Can you work these out from the model? Positions are in its coordinate system, mm. Face numbers are marked on the shaded views. A direction names the side the tool comes from. Give positions to 0.01 mm unless a question says otherwise; leave off trailing zeros. Order: outer loops, then holes, each group sorted by start corner. A loop starts at its lowest first (then second) coordinate and runs counter-clockwise, first axis right, second up. Notation, with made-up numbers: (-18, 28.5) - (8, 28.5) arc R33 cw to (8, 61.5) - close; hole circle Ø1 at (-26, 10). An arc over 180 degrees is marked (long way). Answer as CSV lines item,"result".
```python
from build123d import *

# Parameters (mm, degrees)
BOSS_EXTRUDE1_DEPTH = 8.636


with BuildPart() as part:
    # Sketch1 → Revolve1 (revolve)
    with BuildSketch(Plane.XY):
        Polygon((0, 0), (0, 29.972), (6.477, 29.972), (6.477, 38.354), (11.1125, 38.354), (11.1125, 0), (11.1125, -27.432), (4.5125, -27.432), (4.5125, -8.636), (0, -8.636), align=None)
    revolve(axis=Axis((11.1125, 38.354, 0), (0, -1, 0)))

    # Sketch2 → Boss-Extrude1 (add)
    with BuildSketch(Plane.XZ.offset(8.636)):
        Polygon((23.944109733, 0), (17.528304866, 11.1125), (4.696695134, 11.1125), (-1.719109733, 0), (4.696695134, -11.1125), (17.528304866, -11.1125), align=None)
    extrude(amount=-BOSS_EXTRUDE1_DEPTH)


solid = part.part
```
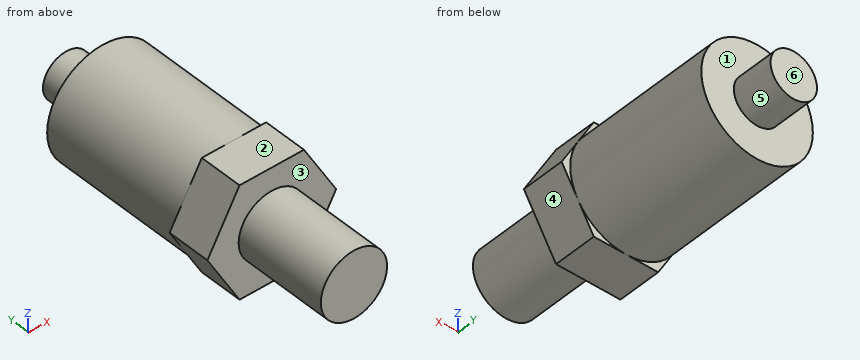
1) I want a section at A-A on z = 2.25. Write out the boundary of the cut face in (x, y), plus the area to 3 significant figures.
Answer block:
outline,"(-0.42, -8.64) - (4.91, -8.64) - (4.91, -27.43) - (17.32, -27.43) - (17.32, -8.64) - (22.65, -8.64) - (22.65, 0) - (21.99, 0) - (21.99, 29.97) - (15.17, 29.97) - (15.17, 38.35) - (7.06, 38.35) - (7.06, 29.97) - (0.23, 29.97) - (0.23, 0) - (-0.42, 0) - close"
area,"1,150 mm2"
2) Which directions (+Z, -Z, +X, -X, +Y, -Y) give clear straight access to the entire face, cutting with the end or side of a thin tool? Please do the marked faces 1, 2 and 3.
Answer block:
face 1,"+Y"
face 2,"+Z, +X, -X, +Y, -Y"
face 3,"-Y"
3) If we mould it in two halves opening along Z, with no side actions, what happens to the marked faces 4, 5 and 6? For each: +Z half, -Z half, draft (parallel to the pull), parting line (faces both ways), or undercut.
Answer block:
face 4,"-Z half"
face 5,"parting line"
face 6,"draft"
4) I want a section at B-B on x = 13. Write out the boundary of the cut face in (y, z), plus the area to 3 significant figures.
Answer block:
outline,"(-27.43, -6.32) - (-8.64, -6.32) - (-8.64, -11.11) - (0, -11.11) - (0, -10.95) - (29.97, -10.95) - (29.97, -4.23) - (38.35, -4.23) - (38.35, 4.23) - (29.97, 4.23) - (29.97, 10.95) - (0, 10.95) - (0, 11.11) - (-8.64, 11.11) - (-8.64, 6.32) - (-27.43, 6.32) - close"
area,"1,160 mm2"
5) I want a section at C-C on y = 5.5. Write out the boundary of the cut face in (x, z) (1 decimal).
Answer block:
outline,"circle Ø22.2 at (11.1, 0)"
6) I want a section at D-D on y = 32. Write out the boundary of the cut face in (x, z), plus the area to 3 significant figures.
Answer block:
outline,"circle Ø9.27 at (11.11, 0)"
area,"67.5 mm2"
7) I'm going to push flat-ended pins straight in: P1, Ø3.5, axis at x = 22, z = 1, coming from the +Y side; P2, Ø2, axis at x = 15.5, y = 22.5, coming from the +Z side; P3, Ø4, axis at y = 9.5, z = -4, coming from the -X side; P4, Ø1.5, axis at x = 1, y = -11, coming from the -Z side. Where does each tip first touch, or does it pass through?
Answer block:
P1,"y = 29.97"
P2,"z = 10.58"
P3,"x = 0.18"
P4,"through"
8) I need wall thicknesses on line 1 along Y through (x, z) = (13.25, 4.75); line 2 along Y through (x, z) = (10, -9.25); line 3 along Z through (x, y) = (10.75, 23). Which ranges of each line are inside material? Lowest first, please. Write a range as [from, to].
Answer block:
line 1,"[-27.43, 29.97]"
line 2,"[-8.64, 29.97]"
line 3,"[-11.11, 11.11]"
